from build123d import *

# Parameters (mm, degrees)
BOSS_EXTRUDE1_DEPTH = 2.54
SKETCH2_W           = 19.05
SKETCH2_H           = 2.54
BOSS_EXTRUDE2_DEPTH = 1.27


with BuildPart() as part:
    # Sketch1 → Boss-Extrude1 (new body)
    with BuildSketch(Plane(origin=(0, 0, 0), x_dir=(1, 0, 0), z_dir=(0, 1, 0))):
        with BuildLine():
            Line((-22.7965, -11.4935), (22.7965, -11.4935))
            ThreePointArc((22.7965, -11.4935), (23.694525612, -11.121525612), (24.0665, -10.2235))
            Line((24.0665, -10.2235), (24.0665, 10.2235))
            ThreePointArc((24.0665, 10.2235), (23.694525612, 11.121525612), (22.7965, 11.4935))
            Line((22.7965, 11.4935), (-22.7965, 11.4935))
            ThreePointArc((-22.7965, 11.4935), (-23.694525612, 11.121525612), (-24.0665, 10.2235))
            Line((-24.0665, 10.2235), (-24.0665, -10.2235))
            ThreePointArc((-24.0665, -10.2235), (-23.694525612, -11.121525612), (-22.7965, -11.4935))
        make_face()
    extrude(amount=-BOSS_EXTRUDE1_DEPTH)

    # Sketch2 → Boss-Extrude2 (add, symmetric)
    with BuildSketch(Plane.XY):
        with Locations((0, 1.27)):
            Rectangle(SKETCH2_W, SKETCH2_H)
    extrude(amount=BOSS_EXTRUDE2_DEPTH, both=True)


solid = part.part
Verification items for the finished model (mm, model axes). A direction names the side the tool comes from. Coordinates: 2 decimals unless noted, no trailing zeros. Write each loop counter-clockwise with the first axis right and the second up, starting at its lowest first coordinate (ties: lowest second). Pieces come first, ordered by that corner, then holes. Notation, with made-up numbers: (44, -26.75) -> (73, -26.75) arc R21 ccw to (73, -13.75) -> close; hole circle Ø9 at (-33.75, -9.75). An arc over 180 degrees is marked (long way). One line per item, written item: value. Start each with the question number.
Q1. Access from +Z, -Z, +X, -X, +Y, -Y to the whole of each face (thin tool, end or side, straight path). Record for faces 1 (the flat face through (9.525, 1, 0)), 2 (the cylindrical face through (23.685, -1.252, 11.131)), 3 (the flat face through (0, 1, 1.27)), 4 (the flat face through (0, 1, -1.27)), 5 (the flat face through (-9.525, 1, 0)).
Q2. Cross-section at A-A on z = 0. Enter the section's corners in (x, y) (1 decimal), and give its area (3 significant figures).
Q3. Cross-section at D-D on x = 12. Enter the section's corners in (y, z).
Q4. Thickness scan on L1, parallel to Y at x = 10, z = 10; L2, parallel to X at y = 0.3, z = 0.75 (3 decimals); L3, parallel to Z at x = 5, y = 0.5. Record the ranges inside material, lowest first. Write a range as from..to.
Q5. Cross-section at C-C on y = 0.8. Enter the section's corners in (x, z) (3 decimals).
Q6. Go/stop test with flat-tipped pins: P1, Ø2, axis at x = 13, z = 5.5, coming from the +Y side; P2, Ø0.8, axis at y = 1.5, z = -0.5, coming from the +X side (3 decimals). Record where each tip stops, or that it passes through.
Q7. Cross-section at B-B on x = -8.5. Enter the section's corners in (y, z).
Checked values:
1. face 1: +Z, -Z, +X, +Y
1. face 2: +Z, +X, +Y, -Y
1. face 3: +Z, +X, -X, +Y
1. face 4: -Z, +X, -X, +Y
1. face 5: +Z, -Z, -X, +Y
2. outline: (-24.1, -2.5) -> (24.1, -2.5) -> (24.1, 0) -> (9.5, 0) -> (9.5, 2.5) -> (-9.5, 2.5) -> (-9.5, 0) -> (-24.1, 0) -> close
2. area: 171 mm²
3. outline: (-2.54, -11.49) -> (0, -11.49) -> (0, 11.49) -> (-2.54, 11.49) -> close
4. L1: y = -2.54..0
4. L2: x = -9.525..9.525
4. L3: z = -1.27..1.27
5. outline: (-9.525, -1.27) -> (9.525, -1.27) -> (9.525, 1.27) -> (-9.525, 1.27) -> close
6. P1: stops at y = 0
6. P2: stops at x = 9.525
7. outline: (-2.54, -11.49) -> (0, -11.49) -> (0, -1.27) -> (2.54, -1.27) -> (2.54, 1.27) -> (0, 1.27) -> (0, 11.49) -> (-2.54, 11.49) -> close
